CAD build for the part. Positions are in the model's coordinates, mm. A direction names the side the tool comes from. Round coordinates to 2 decimals unless told otherwise and drop trailing zeros. Loops run counter-clockwise (first coordinate to the right, second up) from the corner with the lowest first, then second, coordinate; pieces in that order, holes last. Notation, with made-up numbers: M 75,33.5 L 94,33.5 A7 cw 94,38.5 Z; hole C -28.5,6 d1. An arc over 180 degrees is marked long. Use one line per item in the form item = value.
from build123d import *

# Parameters (mm, degrees)
SKETCH_2_R      = 3.85
EXTRUDE_1_DEPTH = 1.5


with BuildPart() as part:
    # 草圖2 → 填料-伸長1 (new body)
    with BuildSketch(Plane(origin=(0, 0, 0), x_dir=(0, 0, -1), z_dir=(1, 0, 0))):
        with BuildLine():
            Line((-86.216124971, 6.090280685), (114.038610046, 6.090280685))
            ThreePointArc((114.038610046, 6.090280685), (120.229892502, 7.285685691), (125.736176674, 10.35843791))
            ThreePointArc((125.736176674, 10.35843791), (147.107034966, 0), (125.736176674, -10.35843791))
            ThreePointArc((125.736176674, -10.35843791), (120.229892502, -7.285685691), (114.038610046, -6.090280685))
            Line((114.038610046, -6.090280685), (-86.216124971, -6.090280685))
            ThreePointArc((-86.216124971, -6.090280685), (-92.407407427, -7.285685691), (-97.913691598, -10.35843791))
            ThreePointArc((-97.913691598, -10.35843791), (-119.284549891, 0), (-97.913691598, 10.35843791))
            ThreePointArc((-97.913691598, 10.35843791), (-92.407407427, 7.285685691), (-86.216124971, 6.090280685))
        make_face()
        with Locations((133.911242538, 0)):
            Circle(SKETCH_2_R, mode=Mode.SUBTRACT)
        with Locations((-106.088757462, 0)):
            Circle(SKETCH_2_R, mode=Mode.SUBTRACT)
    extrude(amount=EXTRUDE_1_DEPTH)


solid = part.part
1. Cut at B-B on x = 0.45. Write the cut outline in (y, z).
Completed:
outline = M -10.36,-125.74 A13.2 ccw long 10.36,-125.74 A19.9 cw 6.09,-114.04 L 6.09,86.22 A19.9 cw 10.36,97.91 A13.2 ccw long -10.36,97.91 A19.9 cw -6.09,86.22 L -6.09,-114.04 A19.9 cw Z; hole C 0,-133.91 d7.7; hole C 0,106.09 d7.7
2. Drop flat-ended pins along their axis: P1, Ø10, axis at y = 0, z = -133.91, coming from the +X side; P2, Ø4, axis at y = -9, z = 80, coming from the -X side. Give the stop position or say it passes through.
Completed:
P1 = 1.5
P2 = through
3. Tool access for faces 1 (the face through (0.74, -0.41, 119.28)), 2 (the face through (0.74, -7.255, 92.324)), 3 (the face through (0.74, 7.316, 92.491)): list every direction of +Z, -Z, +X, -X, +Y, -Y with a clear straight run to the whole face (end or side of a thin tool).
Completed:
face_1 = +X, -X
face_2 = +X, -X, -Y
face_3 = +X, -X, +Y
4. Cut at A-A on y = 0. Write the cut outline in (x, z), and give its area (3 significant figures).
Completed:
outline = M 0,-147.11 L 1.5,-147.11 L 1.5,-137.76 L 0,-137.76 Z; M 0,-130.06 L 1.5,-130.06 L 1.5,102.24 L 0,102.24 Z; M 0,109.94 L 1.5,109.94 L 1.5,119.28 L 0,119.28 Z
area = 376 mm2
5. Probe line 1 along Z through (x, y) = (0.15, -0.75) (3 decimals); line 2 along Y through (x, z) = (0.65, -66); line 3 along Z through (x, y) = (0.65, -2.5). List the from-to ranges inside material, lowest first. Write a range as from..to.
Completed:
line_1 = -147.086..-137.687, -130.135..102.313, 109.865..119.263
line_2 = -6.09..6.09
line_3 = -146.87..-136.84, -130.98..103.16, 109.02..119.05
6. Pull direction Y, two halves, no side cores. Call faces 4 (the face through (0.74, 7.255, -120.147)), 5 (the face through (0.74, 0.169, 109.935)), 6 (the face through (0.74, -7.316, -120.313)): +Y half, -Y half, draft (parallel to the pull), parting line (faces both ways), or undercut.
Completed:
face_4 = +Y half
face_5 = undercut
face_6 = -Y half
7. Cut at C-C on z = 32. Write the cut outline in (x, y), and give its area (3 significant figures).
Completed:
outline = M 0,-6.09 L 1.5,-6.09 L 1.5,6.09 L 0,6.09 Z
area = 18.3 mm2
